Autodesk Inventor part; units mm, degrees
ref_plane "Combination_Module_XY" through (0, 0, 0) normal (1, 0, 0) x (0, 0, -1)
ref_plane "Combination_Module_YZ" through (0, 0, 0) normal (0, 0, -1) x (0, 1, 0)
ref_plane "Combination_Module_ZX" through (0, 0, 0) normal (0, 1, 0) x (1, 0, 0)
sketch "Sketch_1" plane through (0, 0, 0) normal (0, 0, 1) x (1, 0, 0)
  line L0 (24, 0) -> (0, 0)
  line L1 (0, 4) -> (24, 4)
  line L2 (24, 4) -> (24, 6.75)
  arc A0 (24, 6.75) -> (23.25, 7.5) centre (23.25, 6.75) ccw
  line L3 (23.25, 7.5) -> (6, 7.5)
  line L4 (6, 7.5) -> (6, 7.2)
  line L5 (6, 7.2) -> (5, 7.2)
  line L6 (5, 7.2) -> (5, 16)
  line L7 (5, 16) -> (0, 16)
  line L8 (0, 16) -> (0, 4)
revolve "Revolution1" add sketch "Sketch_1" angle 360 about axis through (24, 0, 0) along (1, 0, 0)
sketch "Sketch2" plane through (0, 0, 0) normal (-1, 0, 0) x (0, 0, 1)
  point P0 (0, 12)
hole "Hole1" at (0, 12, 0) direction (1, 0, 0) diameter 3.5 depth 5 counterbore diameter 6 counterbore depth 3.1
sketch "Sketch3" plane through (0, 0, 0) normal (-1, 0, 0) x (0, 0, 1)
  point P0 (0, -12)
hole "Hole2" at (0, -12, 0) direction (1, 0, 0) diameter 3.5 depth 5 counterbore diameter 6 counterbore depth 3.1
sketch "Sketch4" plane through (0, 0, 0) normal (-1, 0, 0) x (0, 0, 1)
  point P0 (-12, 0)
hole "Hole3" at (0, 0, -12) direction (1, 0, 0) diameter 3.5 depth 5 counterbore diameter 6 counterbore depth 3.1
sketch "Sketch5" plane through (0, 0, 0) normal (-1, 0, 0) x (0, 0, 1)
  point P0 (12, 0)
hole "Hole4" at (0, 0, 12) direction (1, 0, 0) diameter 3.5 depth 5 counterbore diameter 6 counterbore depth 3.1
ref_plane "Combination_Module_XY" through (0, 0, 0) normal (1, 0, 0) x (0, 0, -1)
ref_plane "Combination_Module_YZ" through (0, 0, 0) normal (0, 0, -1) x (0, 1, 0)
ref_plane "Combination_Module_ZX" through (0, 0, 0) normal (0, 1, 0) x (1, 0, 0)
properties part number "LHFR-N8" material "鉄、鋳鉄"
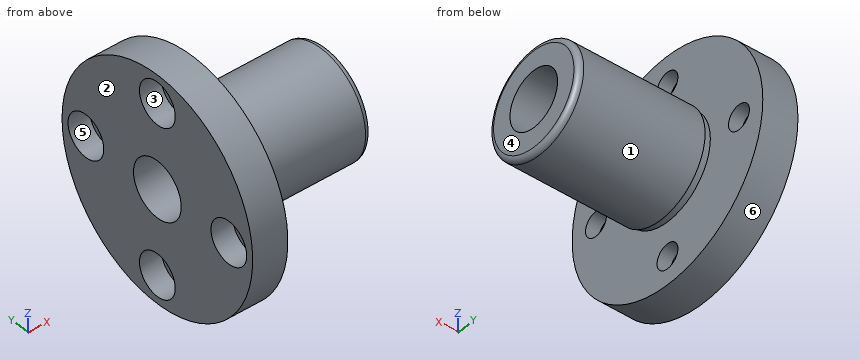
Input: part model. Units: mm. Frame: model coordinates. Face numbers are marked on the shaded views. A direction names the side the tool comes from. Coordinates: 2 decimals unless noted, no trailing zeros. Loops run counter-clockwise (first coordinate to the right, second up) from the corner with the lowest first, then second, coordinate; pieces in that order, holes last. Notation, with made-up numbers: (43.25, 64.25) -> (88.25, 64.25) arc R18 cw to (88.25, 96.25) -> close; hole circle Ø9 at (76, 57.5). An arc over 180 degrees is marked (long way). Write each question's results on one line, items separated by ' | '. Start each with the question number.
Q1. Section C-C, the plane y = -12. Return the cut outline in (x, z), plus the area to 3 significant figures.
Q2. Reachability of the marked faces 1, 2 and 3 from +Z, -Z, +X, -X, +Y, -Y: full face, straight path, thin tool, end or side. Return the list, or none.
Q3. Pin query (flat end, axial travel): pin 1 (10 mm diameter, centred on y = 9, z = -9, fed in from +X); pin 2 (2 mm diameter, centred on x = 16.5, z = -1.5, fed in from -Y); pin 3 (6.5 mm diameter, centred on y = 1, z = -13, fed in from -X); pin 4 (10 mm diameter, centred on x = 5, z = 10.5, fed in from -Y) (3 decimals). Return the tip coordinate at first contact, or that it passes through.
Q4. Pull-direction query (Z, two-part tool) for the marked faces 4, 5 and 6; classes: released by +Z, released by -Z, zero draft, split by the parting line, or undercut.
Q5. Section A-A, the plane z = 0. State how many separate pieces and enclosed holes the cut face has, plus the area to 3 significant figures.
Q6. Ray query, line 1 (Z direction, x = 1.7, y = 0); line 2 (Z direction, x = 3, y = -1.5); line 3 (X direction, y = -8, z = -8.5). Return the intervals inside material, ascending. Write a range as from..to.
Found:
1) outline: (0, -10.58) -> (5, -10.58) -> (5, -1.75) -> (3.1, -1.75) -> (3.1, -3) -> (0, -3) -> close; (0, 3) -> (3.1, 3) -> (3.1, 1.75) -> (5, 1.75) -> (5, 10.58) -> (0, 10.58) -> close | area: 80.6 mm2
2) face 1: +X | face 2: +Z, -Z, -X, +Y, -Y | face 3: -X
3) pin 1: x = 5 | pin 2: y = -7.48 | pin 3: x = 0 | pin 4: y = -15.025
4) face 4: zero draft | face 5: undercut | face 6: split by the parting line
5) separate pieces: 4 | enclosed holes: 0 | area: 202 mm2
6) line 1: -16..-15, -9..-4, 4..9, 15..16 | line 2: -15.93..-14.6, -9.4..-3.71, 3.71..9.4, 14.6..15.93 | line 3: 0..5
